```python
from build123d import *

# Parameters (mm, degrees)
SKETCH1_R                                         = 38.1
SKETCH1_R_2                                       = 31.75
BOSS_EXTRUDE1_DEPTH                               = 2.54
SKETCH2_W                                         = 10.16
SKETCH2_H                                         = 12.7
BOSS_EXTRUDE2_DEPTH                               = 2.54
FILLET1_R                                         = 2.54
SKETCH3_R                                         = 0.635
CUT_EXTRUDE1_DEPTH                                = 3.54
CSK_FOR_2_FLAT_HEAD_MACHINE_SCREW_100_D           = 2.4384
CSK_FOR_2_FLAT_HEAD_MACHINE_SCREW_100_CSINK_D     = 4.3688
CSK_FOR_2_FLAT_HEAD_MACHINE_SCREW_100_CSINK_ANGLE = 100
CIRPATTERN1_COUNT                                 = 3
FILLET1_OF_CIRPATTERN1_R                          = 2.54
SKETCH6_R                                         = 36.9697
SKETCH6_R_2                                       = 34.544
CUT_EXTRUDE3_DEPTH                                = 1.27


with BuildPart() as part:
    # Sketch1 → Boss-Extrude1 (new body)
    with BuildSketch(Plane.XY):
        Circle(SKETCH1_R)
        Circle(SKETCH1_R_2, mode=Mode.SUBTRACT)
    extrude(amount=BOSS_EXTRUDE1_DEPTH)

    # Sketch2 → Boss-Extrude2 (add)
    with BuildSketch(Plane.XY):
        with Locations((38.1, 0)):
            Rectangle(SKETCH2_W, SKETCH2_H)
    boss_extrude2 = extrude(amount=BOSS_EXTRUDE2_DEPTH)

    # Fillet1
    fillet1_edges = [part.edges().sort_by_distance(p)[0] for p in [
        (43.18, 6.35, 1.27),
        (43.18, -6.35, 1.27),
    ]]
    fillet(fillet1_edges, radius=FILLET1_R)

    # Sketch3 → Cut-Extrude1 (cut, through all)
    with BuildSketch(Plane.XY.offset(2.54)):
        with Locations((39.37, 0)):
            Circle(SKETCH3_R)
    cut_extrude1 = extrude(amount=-CUT_EXTRUDE1_DEPTH, mode=Mode.SUBTRACT)

    # CSK for #2 Flat Head Machine Screw (100)1 (through all)
    with Locations(Plane.XY.offset(2.54)):
        with Locations((39.37, 0)):
            csk_for_2_flat_head_machine_screw_100 = CounterSinkHole(CSK_FOR_2_FLAT_HEAD_MACHINE_SCREW_100_D / 2, CSK_FOR_2_FLAT_HEAD_MACHINE_SCREW_100_CSINK_D / 2, counter_sink_angle=CSK_FOR_2_FLAT_HEAD_MACHINE_SCREW_100_CSINK_ANGLE)

    # CirPattern1: Boss-Extrude2, Cut-Extrude1, CSK for #2 Flat Head Machine Screw (100)1 ×3 about axis
    cirpattern1_axis = Axis((0, 0, 0), (0, 0, 1))
    for i in range(1, CIRPATTERN1_COUNT):
        add(boss_extrude2.rotate(cirpattern1_axis, i * 360 / CIRPATTERN1_COUNT))
        add(cut_extrude1.rotate(cirpattern1_axis, i * 360 / CIRPATTERN1_COUNT), mode=Mode.SUBTRACT)
        add(csk_for_2_flat_head_machine_screw_100.rotate(cirpattern1_axis, i * 360 / CIRPATTERN1_COUNT), mode=Mode.SUBTRACT)

    # Fillet1 of CirPattern1
    fillet1_of_cirpattern1_edges = [part.edges().sort_by_distance(p)[0] for p in [
        (-27.089261314, 34.219976935, 1.27),
        (-16.090738686, 40.569976935, 1.27),
        (-16.090738686, -40.569976935, 1.27),
        (-27.089261314, -34.219976935, 1.27),
    ]]
    fillet(fillet1_of_cirpattern1_edges, radius=FILLET1_OF_CIRPATTERN1_R)

    # Sketch6 → Cut-Extrude3 (cut)
    with BuildSketch(Plane(origin=(0, 0, 0), x_dir=(-1, 0, 0), z_dir=(0, 0, -1))):
        Circle(SKETCH6_R)
        Circle(SKETCH6_R_2, mode=Mode.SUBTRACT)
    extrude(amount=-CUT_EXTRUDE3_DEPTH, mode=Mode.SUBTRACT)


solid = part.part
```
Work out the finished part from the listing and answer in its coordinate system (mm). A direction names the side the tool comes from. Coordinates: 2 decimals unless noted, no trailing zeros. Loops run counter-clockwise (first coordinate to the right, second up) from the corner with the lowest first, then second, coordinate; pieces in that order, holes last.
1) Section D-D (y = -12) is taken. Give the vertices of the cut face in (x, z).
Results:
outline: (-36.16, 0) - (-34.97, 0) - (-34.97, 1.27) - (-32.39, 1.27) - (-32.39, 0) - (-29.39, 0) - (-29.39, 2.54) - (-36.16, 2.54) - close; (29.39, 0) - (32.39, 0) - (32.39, 1.27) - (34.97, 1.27) - (34.97, 0) - (36.16, 0) - (36.16, 2.54) - (29.39, 2.54) - close
2) Section B-B (y = 0) is taken. Give the vertices of the cut face in (x, z).
Results:
outline: (-38.1, 0) - (-36.97, 0) - (-36.97, 1.27) - (-34.54, 1.27) - (-34.54, 0) - (-31.75, 0) - (-31.75, 2.54) - (-38.1, 2.54) - close; (31.75, 0) - (34.54, 0) - (34.54, 1.27) - (36.97, 1.27) - (36.97, 0) - (38.15, 0) - (38.15, 1.73) - (37.19, 2.54) - (31.75, 2.54) - close; (40.59, 0) - (43.18, 0) - (43.18, 2.54) - (41.55, 2.54) - (40.59, 1.73) - close
3) For a pull along Y with two mould halves and no side action, classify faces 3 (the flat face through (43.18, 0, 1)), 4 (the cylindrical face through (18.64, -33.23, 1.25)), 5 (the cylindrical face through (-20.34, -33.067, 0.853)) as +Y half, -Y half, draft (parallel to the pull), parting line (faces both ways), or undercut.
Results:
face 3: draft
face 4: -Y half
face 5: undercut
4) Flat-ended cylindrical pins translate along their axes: pin 1 (3 mm diameter, centred on x = 39.37, y = 0, fed in from -Z); pin 2 (1 mm diameter, centred on x = -25, z = 2, fed in from +Y); pin 3 (1.3 mm diameter, centred on x = 39.5, z = 2, fed in from -Y). Find the tip coordinate at first contact, or state that the pin passes through.
Results:
pin 1: stops at z = 0
pin 2: stops at y = 35.71
pin 3: stops at y = -6.35
5) Consider probe 1 along Y at (x, z) = (-25, 2.05); probe 2 along Y at (x, z) = (-4.5, 1); probe 3 along Y at (x, z) = (39.37, 0.85). Determine where each line is inside the solid, lowest interval first.
Results:
probe 1: y = -35.42 to -30.6, -28.75 to -19.57, 19.57 to 28.75, 30.6 to 35.42
probe 2: y = -37.83 to -36.69, -34.25 to -31.43, 31.43 to 34.25, 36.69 to 37.83
probe 3: y = -6.35 to -1.22, 1.22 to 6.35
6) Section A-A (x = 0) is taken. Give the vertices of the cut face in (y, z).
Results:
outline: (-38.1, 0) - (-36.97, 0) - (-36.97, 1.27) - (-34.54, 1.27) - (-34.54, 0) - (-31.75, 0) - (-31.75, 2.54) - (-38.1, 2.54) - close; (31.75, 0) - (34.54, 0) - (34.54, 1.27) - (36.97, 1.27) - (36.97, 0) - (38.1, 0) - (38.1, 2.54) - (31.75, 2.54) - close
7) Section C-C (z = 0.65) is taken. Give the vertices of the cut face in (x, y) (3 decimals).
Results:
outline: circle Ø69.088 at (0, 0); (-25.819, -32.02) arc R2.54 ccw to (-24.89, -35.49) - (-18.29, -39.3) arc R2.54 ccw to (-14.821, -38.37) - (-13.284, -35.709) arc R38.1 ccw to (37.567, -6.35) - (40.64, -6.35) arc R2.54 ccw to (43.18, -3.81) - (43.18, 3.81) arc R2.54 ccw to (40.64, 6.35) - (37.567, 6.35) arc R38.1 ccw to (-13.284, 35.709) - (-14.821, 38.37) arc R2.54 ccw to (-18.29, 39.3) - (-24.89, 35.49) arc R2.54 ccw to (-25.819, 32.02) - (-24.283, 29.359) arc R38.1 ccw to (-24.283, -29.359) - close; hole circle Ø73.939 at (0, 0); hole circle Ø63.5 at (0, 0); hole circle Ø2.438 at (-19.685, -34.095); hole circle Ø2.438 at (-19.685, 34.095); hole circle Ø2.438 at (39.37, 0)
8) For faces 1 (the cylindrical face through (4.5, 34.25, 0.63)), 2 (the cylindrical face through (-16.336, -39.546, 1.288)), determine the directions among +Z, -Z, +X, -X, +Y, -Y from which every point of the face is accessible in a straight line to the end or side of a thin tool.
Results:
face 1: -Z
face 2: +Z, -Z, -Y
